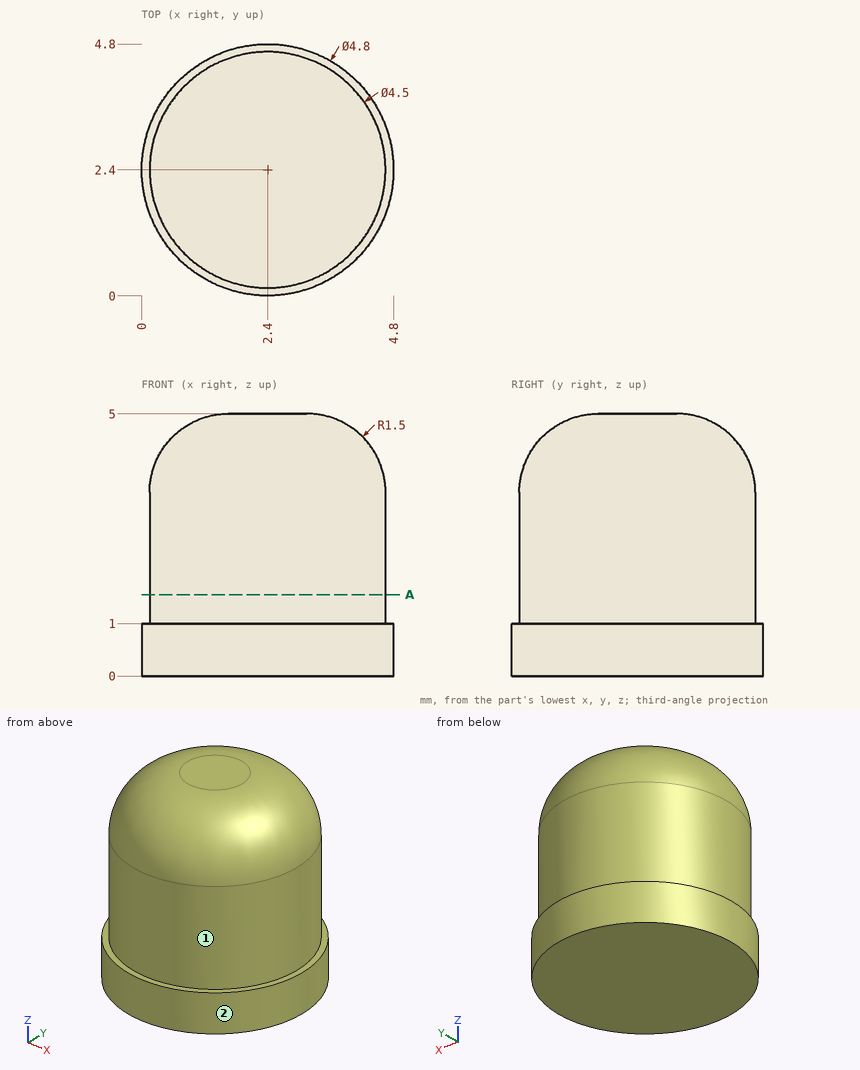
The figure shows three views and two pictorial views of one solid part (mm, origin at its lowest corner). Answer the questions. A direction names the side the tool comes from. Coordinates: 2 decimals unless noted, no trailing zeros. Loops run counter-clockwise (first coordinate to the right, second up) from the corner with the lowest first, then second, coordinate; pieces in that order, holes last. Notation, with made-up numbers: M 22.25,-19.75 L 76.25,-19.75 A27 ccw 76.25,-0.75 Z; hole C 84.25,-19 d3. An arc over 180 degrees is marked long. Use CSV: the item, a comma, the result in double quotes. Start each with the question number.
(1) Find section A-A, the plane z = 1.55. Give the vertices of the cut face in (x, y).
(2) For the marked faces 1 and 2, determine the directions among +Z, -Z, +X, -X, +Y, -Y from which every point of the face is accessible in a straight line to the end or side of a thin tool.
(3) Given pin 1 Ø1.5 at (y, z) = (1, 4.5) entering from +X; pin 2 Ø1 at (y, z) = (2, 3) entering from -X; pin 3 Ø1.5 at (y, z) = (1.5, 3.5) entering from +X (3 decimals), each flat-ended and moving along its own axis, determine where each tip first touches the part or whether it passes through.
(4) Consider line 1 (Z direction, x = 1.6, y = 4.6); line 2 (X direction, y = 2.5, z = 0.85); line 3 (Z direction, x = 2.85, y = 1.7). Determine where each line is inside the solid, lowest interval first.
Recorded:
1,outline,"C 2.4,2.4 d4.5"
2,face 1,"+Z"
2,face 2,"+Z, -Z"
3,pin 1,"stops at x = 4.39"
3,pin 2,"stops at x = 0.15"
3,pin 3,"stops at x = 4.645"
4,line 1,"z = 0 to 1"
4,line 2,"x = 0 to 4.8"
4,line 3,"z = 0 to 5"
